Read the model definition and answer for the solid it produces. Units are mm, in the model's axes. Face numbers are marked on the shaded views. Coordinates: 2 decimals unless noted, no trailing zeros. Loops run counter-clockwise (first coordinate to the right, second up) from the corner with the lowest first, then second, coordinate; pieces in that order, holes last. Notation, with made-up numbers: M 88.25,-1.5 L 138.25,-1.5 A10 ccw 138.25,8.5 Z; hole C 67.25,70 d11. An arc over 180 degrees is marked long. One line per item, written item: value. Start each with the question number.
1. The part is cut by section A-A (x = 6.05). Write down the section's boundary in (y, z).
2. The part is cut by section D-D (z = 10.75). Write down the section's boundary in (x, y) (3 decimals).
3. The part is cut by section B-B (x = 0). Write down the section's boundary in (y, z) (3 decimals), then the cut area to 3 significant figures.
4. Flat-ended cylindrical pins translate along their axes: pin 1 (6 mm diameter, centred on x = -3, z = 10, fed in from -Y); pin 2 (6 mm diameter, centred on x = 4, z = 5, fed in from +Y). Find the tip coordinate at first contact, or state that the pin passes through.
5. The part is cut by section C-C (y = 10.75). Write down the section's boundary in (x, z), then the cut area to 3 significant figures.
6. Consider probe 1 along Y at (x, z) = (-6.05, 0.95); probe 2 along Y at (x, z) = (0, 12) (3 decimals); probe 3 along Z at (x, y) = (2.5, 2.75). Determine where each line is inside the solid, lowest interval first.
7. Determine the mould class of the marked faces 1, 2, 3 and 4 for opening direction X: +X half, -X half, draft (parallel to the pull), parting line (faces both ways), or undercut.
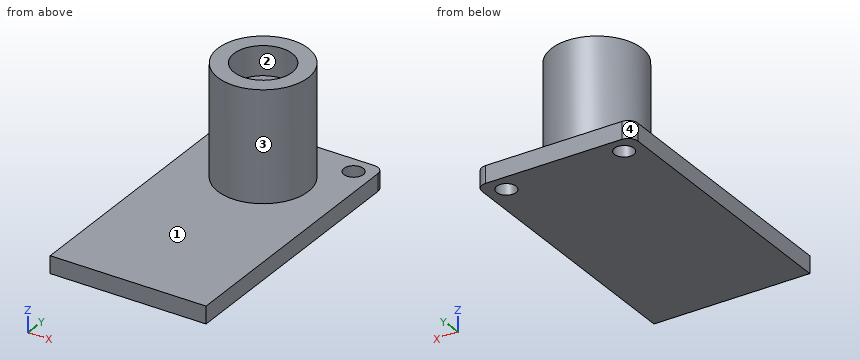
```python
from build123d import *

# Parameters (mm, degrees)
BOSS_EXTRUDE1_DEPTH = 1.78
SKETCH2_R           = 4.655
BOSS_EXTRUDE2_DEPTH = 11.34
SKETCH3_R           = 3
CUT_EXTRUDE1_DEPTH  = 3
SKETCH4_R           = 1
CUT_EXTRUDE2_DEPTH  = 3


with BuildPart() as part:
    # Sketch1 → Boss-Extrude1 (new body)
    with BuildSketch(Plane.XY):
        with BuildLine():
            Line((8.01, -14.14), (-8.01, -14.14))
            Line((-8.01, -14.14), (-8.01, 13.14))
            ThreePointArc((-8.01, 13.14), (-7.717106781, 13.847106781), (-7.01, 14.14))
            Line((-7.01, 14.14), (7.01, 14.14))
            ThreePointArc((7.01, 14.14), (7.717106781, 13.847106781), (8.01, 13.14))
            Line((8.01, 13.14), (8.01, -14.14))
        make_face()
    extrude(amount=BOSS_EXTRUDE1_DEPTH)

    # Sketch2 → Boss-Extrude2 (add)
    with BuildSketch(Plane.XY.offset(1.78)):
        with Locations((0, 7.285)):
            Circle(SKETCH2_R)
    extrude(amount=BOSS_EXTRUDE2_DEPTH)

    # Sketch3 → Cut-Extrude1 (cut)
    with BuildSketch(Plane.XY.offset(13.12)):
        with Locations((0, 7.285)):
            Circle(SKETCH3_R)
    extrude(amount=-CUT_EXTRUDE1_DEPTH, mode=Mode.SUBTRACT)

    # Sketch4 → Cut-Extrude2 (cut)
    with BuildSketch(Plane.XY.offset(1.78)):
        with Locations((6.05, 12.299860012)):
            Circle(SKETCH4_R)
        with Locations((-6.05, 12.299860012)):
            Circle(SKETCH4_R)
    extrude(amount=-CUT_EXTRUDE2_DEPTH, mode=Mode.SUBTRACT)


solid = part.part
```
Answer block:
1. outline: M -14.14,0 L 11.3,0 L 11.3,1.78 L -14.14,1.78 Z; M 13.3,0 L 14.14,0 L 14.14,1.78 L 13.3,1.78 Z
2. outline: C 0,7.285 d9.31; hole C 0,7.285 d6
3. outline: M -14.14,0 L 14.14,0 L 14.14,1.78 L 11.94,1.78 L 11.94,13.12 L 10.285,13.12 L 10.285,10.12 L 4.285,10.12 L 4.285,13.12 L 2.63,13.12 L 2.63,1.78 L -14.14,1.78 Z
3. area: 138 mm2
4. pin 1: stops at y = 2.63
4. pin 2: stops at y = 11.83
5. outline: M -8.01,0 L 8.01,0 L 8.01,1.78 L 3.11,1.78 L 3.11,13.12 L -3.11,13.12 L -3.11,1.78 L -8.01,1.78 Z
5. area: 99.0 mm2
6. probe 1: y = -14.14 to 11.3, 13.3 to 14.14
6. probe 2: y = 2.63 to 4.285, 10.285 to 11.94
6. probe 3: z = 0 to 1.78
7. face 1: draft
7. face 2: undercut
7. face 3: parting line
7. face 4: -X half
